Design review of the part built by this model. Coordinates are the model's own, in mm. Face numbers are marked on the shaded views. A direction names the side the tool comes from. Give positions to 0.01 mm unless a question says otherwise; leave off trailing zeros. Write each loop counter-clockwise with the first axis right and the second up, starting at its lowest first coordinate (ties: lowest second). Pieces come first, ordered by that corner, then holes.
Autodesk Inventor part; units mm, degrees
ref_plane "YZ Plane" through (0, 0, 0) normal (1, 0, 0) x (0, 1, 0)
ref_plane "XZ Plane" through (0, 0, 0) normal (0, 1, 0) x (-1, 0, 0)
ref_plane "XY Plane" through (0, 0, 0) normal (0, 0, 1) x (1, 0, 0)
sketch "Sketch1" plane through (0, 0, 0) normal (0, 0, 1) x (1, 0, 0)
  line L0 (23.75, 0.7) -> (25, 0.7)
  line L1 (25, 0.7) -> (25, 0)
  line L2 (25, 0) -> (32.5, 0)
  line L3 (32.5, 0) -> (48, 15.5)
  line L4 (48, 15.5) -> (48, 57.5)
  line L5 (48, 57.5) -> (60, 57.5)
  line L6 (60, 57.5) -> (60, 87.5)
  line L7 (60, 87.5) -> (40, 87.5)
  line L8 (40, 87.5) -> (40, 20)
  line L9 (40, 20) -> (35.81, 20)
  line L10 (35.81, 20) -> (23.75, 0.7)
  line L11 (0, 0) -> (0, 69.5074) construction
  line L12 (50, 87.5) -> (50, 86.5)
  line L13 (50, 86.5) -> (60, 86.5)
  line L14 (48, 57.5) -> (48, 59.8)
  line L15 (48, 59.8) -> (52, 59.8)
  line L16 (52, 59.8) -> (52, 57.5)
  line L17 (60, 78.5) -> (48, 78.5)
  line L18 (48, 78.5) -> (48, 65.8)
  line L19 (48, 65.8) -> (60, 65.8)
  dimension "d0" = 135
  dimension "d2" = 80
  dimension "d3" = 50
  dimension "d4" = 47.5
  dimension "d5" = 65
  dimension "d6" = 20
  dimension "d9" = 30
  dimension "d10" = 120
  dimension "d11" = 0.7
  dimension "d13" = 122
  dimension "d26" = 1
  dimension "d27" = 100
  dimension "d28" = 96
  dimension "d29" = 4
  dimension "d30" = 2.3
  dimension "d31" = 87.5
  dimension "d32" = 6
  dimension "d33" = 8
revolve "Revolution1" add sketch "Sketch1" angle 360 about axis through (0, 0, 0) along (0, 1, 0) contours L10 L9 L8 L7 L12 L13 L6 L17 L18 L19 L5 L16 L15 L14 L4 L3 L2 L1 L0
sketch "Sketch2" plane through (0, 86.5, 0) normal (0, 1, 0) x (1, 0, 0)
  circle A0 centre (55, 0) radius 4
  point P0 (0, 0)
  dimension "d14" = 55
  dimension "d25" = 8
hole "Hole1" at (55, 86.5, 0) direction (0, -1, 0) diameter 4.917 depth 8
pattern_circular "Circular Pattern1" count 8 over 360 about axis through (0, 37.65, 0) along (0, -1, 0) of "Hole1"
chamfer "Chamfer1" distance 0.5 angle 45 3 edges at (-60, 65.8, 0) (-60, 57.5, 0) (-60, 78.5, 0)
sketch "Sketch3" plane through (0, 0, 0) normal (0, -1, 0) x (1, 0, 0)
  point P0 (0, 0)
  point P1 (29.5, 0)
  dimension "d37" = 29.5
hole "Hole2" at (29.5, 0, 0) direction (0, 1, 0) diameter 1.567 depth 5 tip angle 118
pattern_circular "Circular Pattern2" count 4 over 360 about axis through (0, 37.65, 0) along (0, -1, 0) of "Hole2"
properties part number "003" material "Stainless Steel, 440C"
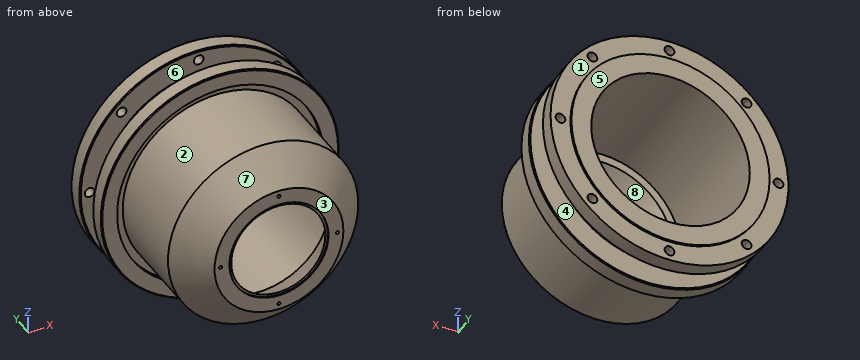
(1) Mouldability with a two-part tool opening along Z and no side actions: class the marked faces 6, 7 and 8 as pulls with the +Z half, pulls with the -Z half, needs draft (parallel to the pull), parting line crosses it, or undercut.
Resolved:
face 6: needs draft
face 7: parting line crosses it
face 8: undercut
(2) Clearance check with flat-ended pins moving along their axes: P1, Ø6, axis at x = 33, y = 63.5, coming from the -Z side; P2, Ø2, axis at x = -29.5, z = 0, coming from the +Y side; P3, Ø4.5, axis at x = 0, z = 55, coming from the -Y side. State where each tip first meets the part, or that it passes through.
Resolved:
P1: stops at z = -51.96
P2: stops at y = 11.5
P3: stops at y = 57.5
(3) Consider section B-B, the plane x = -55. Give the number of separate pieces and of enclosed holes in the cut face, then the cut area to 3 significant figures.
Resolved:
separate pieces: 3
enclosed holes: 0
area: 740 mm2
(4) Tool access review of the marked faces 1, 2, 3, 4 and 5: name each direction out of +Z, -Z, +X, -X, +Y, -Y from which nothing blocks a thin tool from reaching the whole face with its end or side.
Resolved:
face 1: +Y
face 2: -Y
face 3: +Z, -Z, +X, -X, -Y
face 4: none
face 5: +Z, -Z, +X, -X, +Y
(5) Consider section A-A, the plane y = 37. Give the boundary of the cut face in (x, z).
Resolved:
outline: circle Ø96 at (0, 0); hole circle Ø80 at (0, 0)
(6) To check wall thickness, follow L1, parallel to Z at x = 0, y = 58; L2, parallel to Y at x = -53.5, z = 11; L3, parallel to Y at x = 39, z = 29. State the ranges of each line that lie inside material, in increasing order.
Resolved:
L1: z = -60 to -52, -48 to -40, 40 to 48, 52 to 60
L2: y = 57.5 to 65.8, 78.5 to 86.5
L3: y = 59.8 to 65.8, 78.5 to 87.5
